Design review of the part built by this model. Coordinates are the model's own, in mm. A direction names the side the tool comes from. Coordinates: 2 decimals unless noted, no trailing zeros. Loops run counter-clockwise (first coordinate to the right, second up) from the corner with the lowest first, then second, coordinate; pieces in that order, holes last. Notation, with made-up numbers: M 69,77.5 L 86,77.5 A26 ccw 86,105.5 Z; hole C 23.25,-8 d11. An arc over 180 degrees is marked long. One line per item, written item: value.
```python
from build123d import *

# Parameters (mm, degrees)
TRIANGULAR_PRISM_DEPTH = 170
SKETCH5_W              = 20.831302692
SKETCH5_H              = 63.48520277
SKETCH5_W_2            = 25.650693989
SKETCH5_H_2            = 114.24619151
CUT_EXTRUDE1_DEPTH     = 100


with BuildPart() as part:
    # Sketch2 → Pyramid section 0
    with BuildSketch(Plane(origin=(0, 85, 0), x_dir=(-1, 0, 0), z_dir=(0, 1, 0))):
        Polygon((59.282032303, 57.320508076), (7.320508076, 27.320508076), (-22.679491924, 79.282032303), (29.282032303, 109.282032303), align=None)
    # Sketch1 → Pyramid section 1
    with BuildSketch(Plane(origin=(0, 0, 0), x_dir=(1, 0, 0), z_dir=(0, 1, 0))):
        Polygon((0, 0), (-86.602540378, -50), (-36.602540378, -136.602540378), (50, -86.602540378), align=None)
    loft()

    # Sketch4 → Triangular Prism (add)
    with BuildSketch(Plane(origin=(-76.471967598, -27.833519961, 0), x_dir=(0, 0, -1), z_dir=(0.939692621, 0.342020143, 0))):
        Polygon((-97.955549577, 29.619813273), (-40, 45.148955979), (-82.426406871, 87.57536285), align=None)
    extrude(amount=TRIANGULAR_PRISM_DEPTH)

    # Sketch5 → Cut-Extrude1 (cut)
    with BuildSketch(Plane.XY):
        with Locations((-97.018191724, 31.742601385)):
            Rectangle(SKETCH5_W, SKETCH5_H)
        with Locations((62.825346995, 57.123095755)):
            Rectangle(SKETCH5_W_2, SKETCH5_H_2)
    extrude(amount=CUT_EXTRUDE1_DEPTH, mode=Mode.SUBTRACT)


solid = part.part
```
(1) Mouldability with a two-part tool opening along Y and no side actions: class faces 4 (the flat face through (31.06, 74.1, 90.08)), 5 (the flat face through (-86.603, 24, 75)), 6 (the flat face through (-75.04, 10.52, 75.82)) as released by +Y, released by -Y, zero draft, split by the parting line, or undercut.
Reply:
face 4: released by +Y
face 5: zero draft
face 6: undercut
(2) Tool access review of faces 1 (the flat face through (28.6, 80.7, 60.9)), 2 (the flat face through (-73.179, 43.67, 60.916)), 3 (the flat face through (-19, 0, 67)): name each direction out of +Z, -Z, +X, -X, +Y, -Y from which nothing blocks a thin tool from reaching the whole face with its end or side.
Reply:
face 1: -Z, +Y
face 2: -X, +Y
face 3: +Z, -Z, +X, -X, -Y
(3) We need section A-A on y = 98. State the section outline as (x, z) points, then the cut area to 3 significant figures.
Reply:
outline: M 13.2,82.43 L 50,69.84 L 50,85.8 Z
area: 294 mm2
(4) To check wall thickness, follow line 1 along Y through (x, z) = (-12.5, 34.5); line 2 along X through (y, z) = (47, 30); line 3 along Z through (x, y) = (-9.5, 27). State the ranges of each line that lie inside material, in increasing order. Write a range as [from, to].
Reply:
line 1: y = [0, 85]
line 2: x = [-29.84, 4.55]
line 3: z = [12.82, 113.62]
(5) Insertion check: pin 1 (2 mm diameter, centred on y = 24.5, z = 75, fed in from +X); pin 2 (3 mm diameter, centred on y = 19.5, z = 39.5, fed in from +X); pin 3 (5 mm diameter, centred on x = -50.5, y = 37.5, fed in from -Z). Each pin has a flat end and moves straight along its axis. Give the tip position at first contact, or say it passes through.
Reply:
pin 1: stops at x = 37.28
pin 2: stops at x = 18.46
pin 3: stops at z = 37.75
